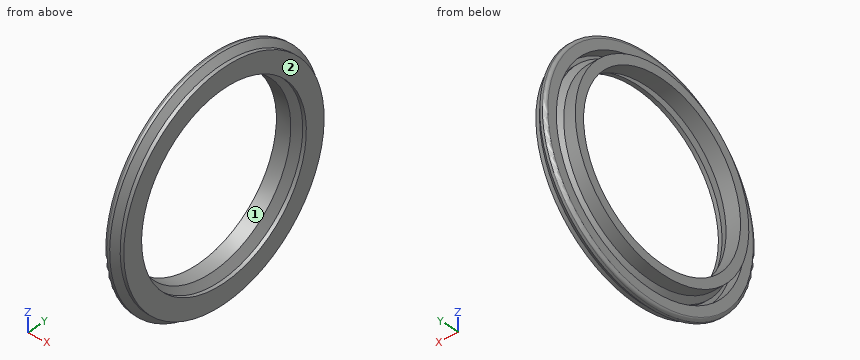
from build123d import *

# Parameters (mm, degrees)
FILLET1_R = 1


with BuildPart() as part:
    # Sketch1 → Revolve1 (revolve)
    with BuildSketch(Plane.XY, mode=Mode.PRIVATE) as revolve1_sk:
        with BuildLine():
            Line((-1.25, 38.305), (-3.125, 40.25))
            Line((-3.125, 40.25), (-5, 40.25))
            Line((-5, 40.25), (-5, 36))
            Line((-5, 36), (-1.25, 36))
            Line((-1.25, 36), (-1.25, 34.59))
            Line((-1.25, 34.59), (-2.48375, 34.59))
            Line((-2.48375, 34.59), (-4.660938533, 32.101784534))
            Line((-4.660938533, 32.101784534), (-5, 33.18))
            Line((-5, 33.18), (-9, 33.18))
            Line((-9, 33.18), (-9, 30))
            Line((-9, 30), (-4, 30))
            Line((-4, 30), (-1.342891128, 34.434956263))
            ThreePointArc((-1.342891128, 34.434956263), (-1.286668766, 34.457448986), (-1.25, 34.409258964))
            Line((-1.25, 34.409258964), (-1.25, 31.5))
            Line((-1.25, 31.5), (0, 31.5))
            Line((0, 31.5), (0, 38.305))
            Line((0, 38.305), (-1.25, 38.305))
        make_face()
    revolve(revolve1_sk.sketch.rotate(Axis((-9, 0, 0), (1, 0, 0)), 270), axis=Axis((-9, 0, 0), (1, 0, 0)))

    # Fillet1
    fillet1_edges = [part.edges().sort_by_distance(p)[0] for p in [
        (-5, 0, 40.25),
    ]]
    fillet(fillet1_edges, radius=FILLET1_R)


solid = part.part
Source: CAD feature listing. Evaluate the final solid. Frame: model axes, mm. Face numbers are marked on the shaded views. Give positions to 0.01 mm unless a question says otherwise; leave off trailing zeros. Return JSON: item names as keys, results as strings. Group by question number.
1) Draft query along Y for the marked faces 1 and 2. Return one class per face: released by +Y, released by -Y, zero draft, split by the parting line, or undercut.
2) Ray query, L1, parallel to Y at x = -2.25, z = -7.5; L2, parallel to Y at x = -0.8, z = 0 (3 decimals); L3, parallel to X at y = 14, z = 30. Return the intervals inside material, ascending.
3) First-contact query: pin 1 Ø1.5 at (x, z) = (-3, 10.5) entering from -Y; pin 2 Ø2 at (x, y) = (-1, 11.5) entering from -Z; pin 3 Ø21.5 at (y, z) = (-12, 12) entering from -X; pin 4 Ø4 at (x, y) = (-3.5, -32) entering from -Z. Flat tips, straight axial feed; report the tip coordinate or a pass-through.
Data:
{
 "1": {"face 1": "undercut", "face 2": "zero draft"},
 "2": {"L1": "y = -38.62 to -35.21, -33.77 to -32.06, 32.06 to 33.77, 35.21 to 38.62", "L2": "y = -38.305 to -31.5, 31.5 to 38.305", "L3": "x = -9 to -4.98, -3.78 to -2.14, -1.25 to 0"},
 "3": {"pin 1": "stops at y = -39.05", "pin 2": "stops at z = -37.39", "pin 3": "passes through", "pin 4": "stops at z = -26.83"}
}
